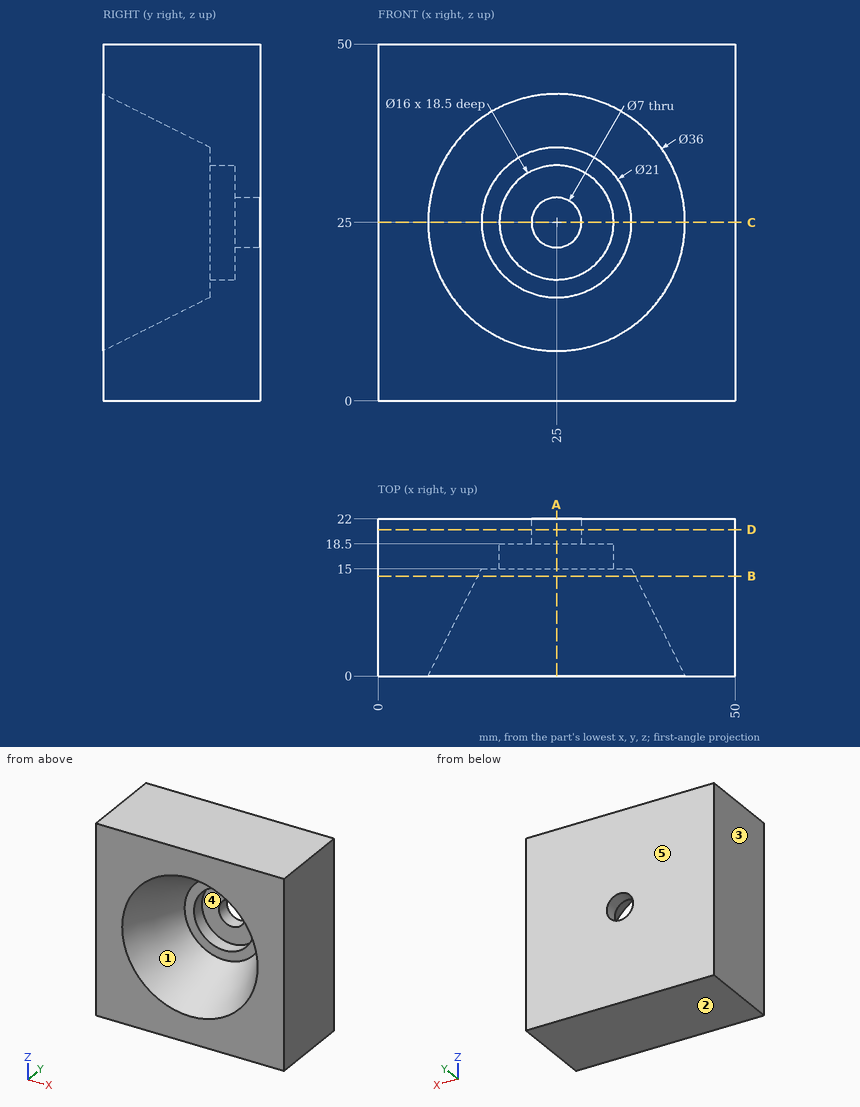
Design review of the part shown in the three views and the two pictorial views. Dimensions are in mm from the part's minimum x, y and z. A direction names the side the tool comes from. Round coordinates to 2 decimals unless told otherwise and drop trailing zeros. Order: outer loops, then holes, each group sorted by start corner. A loop starts at its lowest first (then second) coordinate and runs counter-clockwise, first axis right, second up. Notation, with made-up numbers: (81.5, -2.5) - (128.5, -2.5) arc R29 cw to (128.5, 32.5) - close; hole circle Ø4 at (14.25, 86). An arc over 180 degrees is marked (long way). One line per question, with ' | ' between items.
Item 1: Draft analysis for pull direction X (two halves, no side actions). For the marked faces 1, 2 and 3, state which applies: +X half, -X half, draft (parallel to the pull), parting line (faces both ways), or undercut.
Checks:
face 1: undercut | face 2: draft | face 3: -X half
Item 2: Take a section at C-C, the plane z = 25. Write out the cut boundary in (x, y).
Checks:
outline: (0, 0) - (7, 0) - (14.5, 15) - (17, 15) - (17, 18.5) - (21.5, 18.5) - (21.5, 22) - (0, 22) - close; (28.5, 18.5) - (33, 18.5) - (33, 15) - (35.5, 15) - (43, 0) - (50, 0) - (50, 22) - (28.5, 22) - close
Item 3: Machinability: for the marked faces 4 and 5, which of the approach directions +Z, -Z, +X, -X, +Y, -Y give a long, thin tool a straight path to every point of the face, cutting with its end or side? Answer none if there is none.
Checks:
face 4: -Y | face 5: +Z, -Z, +X, -X, +Y
Item 4: Take a section at B-B, the plane y = 14. Write out the cut boundary in (x, z).
Checks:
outline: (0, 0) - (50, 0) - (50, 50) - (0, 50) - close; hole circle Ø22 at (25, 25)
Item 5: Take a section at D-D, the plane y = 20.5. Write out the cut boundary in (x, z), then the cut area to 3 significant figures.
Checks:
outline: (0, 0) - (50, 0) - (50, 50) - (0, 50) - close; hole circle Ø7 at (25, 25) | area: 2,460 mm²
Item 6: For P1, Ø4, axis at x = 25, z = 25, coming from the -Y side; P2, Ø18.5, axis at x = 25, z = 25, coming from the -Y side; P3, Ø13, axis at x = 28.5, z = 21.5, coming from the -Y side, all flat-tipped, find the tip position at first contact; note any pin that passes through.
Checks:
P1: through | P2: y = 15 | P3: y = 13.1
Item 7: Take a section at A-A, the plane x = 25. Write out the cut boundary in (y, z).
Checks:
outline: (0, 0) - (22, 0) - (22, 21.5) - (18.5, 21.5) - (18.5, 17) - (15, 17) - (15, 14.5) - (0, 7) - close; (0, 43) - (15, 35.5) - (15, 33) - (18.5, 33) - (18.5, 28.5) - (22, 28.5) - (22, 50) - (0, 50) - close
Item 8: Wall thickness on line 1 (Z direction, x = 25, y = 17.2); line 2 (Z direction, x = 25, y = 20.5): over which ranges is each line inside the solid? List them lowest first. Write a range as [from, to].
Checks:
line 1: [0, 17], [33, 50] | line 2: [0, 21.5], [28.5, 50]
